The listing builds one solid part. Answer for the finished solid, in the listing's coordinates (mm). Face numbers are marked on the shaded views. A direction names the side the tool comes from. Give positions to 0.01 mm unless a question says otherwise; leave off trailing zeros. Write each loop counter-clockwise with the first axis right and the second up, starting at its lowest first coordinate (ties: lowest second). Pieces come first, ordered by that corner, then holes. Notation, with made-up numbers: M 58.25,-40 L 79.25,-40 A9 ccw 79.25,-28 Z; hole C 77.25,-11 d2. An arc over 180 degrees is marked long. Answer as a JSON object with one key per item and string values.
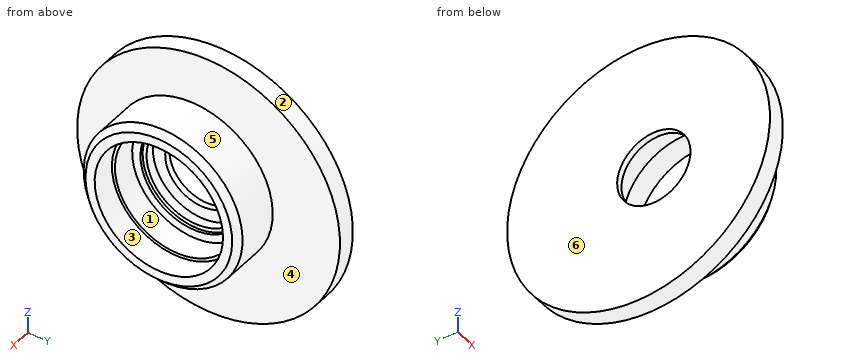
```python
from build123d import *

# Parameters (mm, degrees)
ESQUISSE2_R        = 43
ESQUISSE2_R_2      = 17.284931715
BOSS_EXTRU_1_DEPTH = 6


with BuildPart() as part:
    # Esquisse1 → Base-R_volution (revolve)
    with BuildSketch(Plane.XY, mode=Mode.PRIVATE) as base_r_volution_sk:
        Polygon((0, 12), (0, 26), (20, 26), (22, 24), (22, 21), (14, 21), (14, 20), (5, 20), (5, 16), (2, 16), (2, 12), align=None)
    revolve(base_r_volution_sk.sketch.rotate(Axis((-4.169000368, 0, 0), (1, 0, 0)), 90), axis=Axis((-4.169000368, 0, 0), (1, 0, 0)))

    # Esquisse2 → Boss.-Extru.1 (add)
    with BuildSketch(Plane.ZY):
        with Locations((0, 5)):
            Circle(ESQUISSE2_R)
        Circle(ESQUISSE2_R_2, mode=Mode.SUBTRACT)
    extrude(amount=-BOSS_EXTRU_1_DEPTH)


solid = part.part
```
1. The mould has two halves that part along Y. Classify the marked faces 1, 2, 3 and 4: released by +Y, released by -Y, zero draft, split by the parting line, or undercut.
Verdict:
{"face 1": "undercut", "face 2": "split by the parting line", "face 3": "undercut", "face 4": "zero draft"}
2. A cutting plane is placed at C-C, the plane z = -30.5. Give the vertices of the cut face in (x, y).
Verdict:
{"outline": "M 0,-25.31 L 6,-25.31 L 6,35.31 L 0,35.31 Z"}
3. Flat-ended cylindrical pins translate along their axes: pin 1 (3 mm diameter, centred on x = 11, z = -11.5, fed in from -Y); pin 2 (8 mm diameter, centred on y = 39, z = 0.5, fed in from +X); pin 3 (12 mm diameter, centred on x = 16.5, y = 5, fed in from +Z). Find the tip coordinate at first contact, or state that the pin passes through.
Verdict:
{"pin 1": "stops at y = -24", "pin 2": "stops at x = 6", "pin 3": "stops at z = 26"}
4. For the marked faces 5 and 6, determine the directions among +Z, -Z, +X, -X, +Y, -Y from which every point of the face is accessible in a straight line to the end or side of a thin tool.
Verdict:
{"face 5": "+X", "face 6": "+Z, -Z, -X, +Y, -Y"}
5. A cutting plane is placed at D-D, the plane y = 35.5. Give the vertices of the cut face in (x, z), plus the area to 3 significant figures.
Verdict:
{"outline": "M 0,-30.31 L 6,-30.31 L 6,30.31 L 0,30.31 Z", "area": "364 mm2"}
6. Consider line 1 along Y through (x, z) = (12.5, 0); line 2 along Y through (x, z) = (3.5, 0.5); line 3 along X through (y, z) = (24, -36). Determine where each line is inside the solid, lowest interval first.
Verdict:
{"line 1": "y = -26 to -20, 20 to 26", "line 2": "y = -38 to -15.99, 15.99 to 48", "line 3": "x = 0 to 6"}
